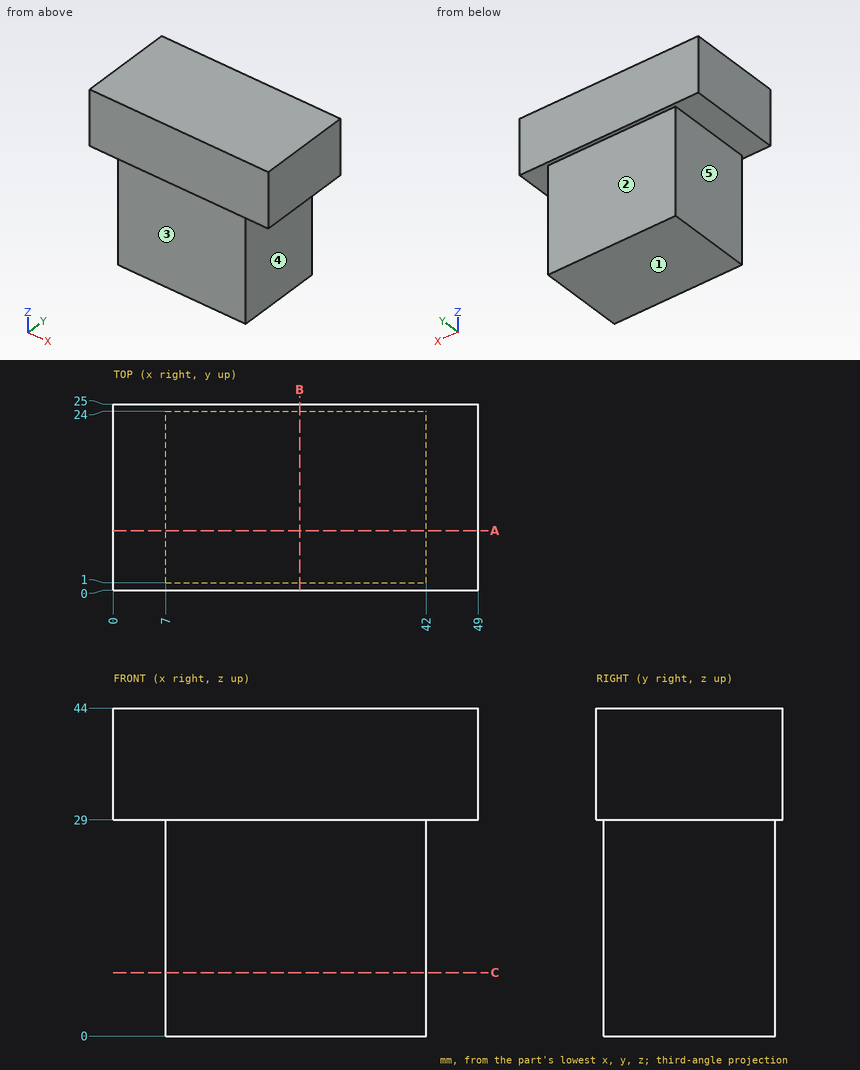
Here's the drawing with two shaded views (mm, measured from the low corner). I have some questions. A direction names the side the tool comes from. Coordinates: 2 decimals unless noted, no trailing zeros. Order: outer loops, then holes, each group sorted by start corner. A loop starts at its lowest first (then second) coordinate and runs counter-clockwise, first axis right, second up.
Q1. Will these pins go through, and if not, where does the flat tip stop? pin 1 (7 mm diameter, centred on y = 7, z = 20, fed in from -X); pin 2 (11.5 mm diameter, centred on y = 17.5, z = 20, fed in from +X); pin 3 (2 mm diameter, centred on x = 39.5, z = 21, fed in from +Y); pin 4 (1.5 mm diameter, centred on x = 5, z = 25, fed in from +Y) (1 decimal).
Q2. Please list where these lines run through material, in increasing order: L1, parallel to X at y = 4.5, z = 18.5; L2, parallel to Y at x = 23, z = 17.5; L3, parallel to Z at x = 43, y = 17.25.
Q3. Suppose I cut it at C-C on z = 8.5. Please give me the cut outline in (x, y).
Q4. Suppose I cut it at B-B on x = 25. Please give me the cut outline in (y, z).
Q5. Suppose I cut it at A-A on y = 8. Please give me the cut outline in (x, z), and give its area (3 significant figures).
Q6. Which directions (+Z, -Z, +X, -X, +Y, -Y) give clear straight access to the entire face, cutting with the end or side of a thin tool? Please do the marked faces 1, 2, 3, 4 and 5.
Answer:
1. pin 1: stops at x = 7
1. pin 2: stops at x = 42
1. pin 3: stops at y = 24
1. pin 4: passes through
2. L1: x = 7 to 42
2. L2: y = 1 to 24
2. L3: z = 29 to 44
3. outline: (7, 1) - (42, 1) - (42, 24) - (7, 24) - close
4. outline: (0, 29) - (1, 29) - (1, 0) - (24, 0) - (24, 29) - (25, 29) - (25, 44) - (0, 44) - close
5. outline: (0, 29) - (7, 29) - (7, 0) - (42, 0) - (42, 29) - (49, 29) - (49, 44) - (0, 44) - close
5. area: 1,750 mm2
6. face 1: -Z, +X, -X, +Y, -Y
6. face 2: -Z, +X, -X, +Y
6. face 3: -Z, +X, -X, -Y
6. face 4: -Z, +X, +Y, -Y
6. face 5: -Z, -X, +Y, -Y
